The listing builds one solid part. Answer for the finished solid, in the listing's coordinates (mm). A direction names the side the tool comes from. Give positions to 0.01 mm unless a question says otherwise; leave off trailing zeros. Write each loop counter-clockwise with the first axis right and the second up, starting at its lowest first coordinate (ties: lowest second). Pieces come first, ordered by that corner, then holes. Notation, with made-up numbers: (60, -16) - (110, -16) arc R20 cw to (110, 20) - close; hole circle Ø10 at (-17, -13.5). An arc over 180 degrees is marked (long way). Return JSON: item names as keys, results as strings.
Autodesk Inventor part; units mm, degrees
ref_plane "YZ Plane" through (0, 0, 0) normal (1, 0, 0) x (0, 1, 0)
ref_plane "XZ Plane" through (0, 0, 0) normal (0, 1, 0) x (-1, 0, 0)
ref_plane "XY Plane" through (0, 0, 0) normal (0, 0, 1) x (1, 0, 0)
sketch "Skizze1" plane through (0, 0, 0) normal (0, 1, 0) x (-1, 0, 0)
  line L0 (25, -25) -> (-25, -25)
  line L1 (-25, -25) -> (-25, 25)
  line L2 (-25, 25) -> (25, 25)
  line L3 (25, 25) -> (25, -25)
  line L4 (25, -25) -> (-25, 25) construction
  line L5 (-25, -25) -> (25, 25) construction
  point P0 (0, 0)
  dimension "d0" = 50
  dimension "d1" = 50
extrude "Extrusion1" add sketch "Skizze1" along normal blind 6
sketch "Skizze2" plane through (0, 0, 0) normal (0, -1, 0) x (1, 0, 0)
  circle A0 centre (-15.75, 15.75) radius 4.25
  circle A1 centre (15.75, 15.75) radius 4.25
  circle A2 centre (15.75, -15.75) radius 4.25
  circle A3 centre (-15.75, -15.75) radius 4.25
  line L0 (-35, 0) -> (35, 0)
  line L1 (0, 35) -> (0, -35)
  point P0 (0, 0)
  dimension "d4" = 31.5
  dimension "d5" = 31.5
  dimension "d6" = 31.5
  dimension "d7" = 31.5
  dimension "d8" = 15.75
  dimension "d9" = 15.75
  dimension "d10" = 15.75
  dimension "d11" = 15.75
  dimension "d12" = 8.5
  dimension "d13" = 8.5
  dimension "d14" = 8.5
  dimension "d15" = 8.5
extrude "Extrusion2" add sketch "Skizze2" along normal blind 1
sketch "Skizze3" plane through (-15.75, -1, 15.75) normal (0, -1, 0) x (1, 0, 0)
  circle A0 centre (0, 0) radius 4.25
  circle A1 centre (0, 0) radius 1.75
  circle A2 centre (31.5, 0) radius 4.25
  circle A3 centre (31.5, 0) radius 1.75
  circle A4 centre (31.5, -31.5) radius 4.25
  circle A5 centre (31.5, -31.5) radius 1.75
  circle A6 centre (0, -31.5) radius 4.25
  circle A7 centre (0, -31.5) radius 1.75
  point P0 (15.75, -15.75)
  dimension "d18" = 3.5
  dimension "d19" = 3.5
  dimension "d20" = 3.5
  dimension "d21" = 3.5
extrude "Extrusion3" cut sketch "Skizze3" against normal blind 13 contours A1 | A3 | A5 | A7
sketch "Skizze4" plane through (0, 0, 0) normal (0, -1, 0) x (1, 0, 0)
  circle A0 centre (-15, 0) radius 1.5
  circle A1 centre (15, 0) radius 1.5
  line L0 (0, 35) -> (0, -35)
  point P0 (0, 0)
  dimension "d24" = 30
  dimension "d25" = 15
  dimension "d26" = 3
  dimension "d27" = 3
extrude "Extrusion4" cut sketch "Skizze4" against normal blind 13
sketch "Skizze7" plane through (0, 6, 0) normal (0, 1, 0) x (1, 0, 0)
  circle A0 centre (15, 0) radius 1.5
  circle A1 centre (15, 0) radius 3
  circle A2 centre (-15, 0) radius 1.5
  circle A3 centre (-15, 0) radius 3
  point P0 (0, 0)
  dimension "d39" = 6
  dimension "d40" = 6
extrude "Extrusion5" cut sketch "Skizze7" against normal blind 4 contours A0 | A1 | A2 | A3
chamfer "Fase1" distance 1 angle 45 2 edges at (12, 2, 0) (-18, 2, 0)
equation "\"d8\" = 0.5 * d6"
equation "\"d9\" = 0.5 * d7"
equation "\"d10\" = 0.5 * d5"
equation "\"d11\" = 0.5 * d4"
equation "\"d25\" = 0.5 * d24"
properties part number "Lagerhalterung"
Item 1: The mould has two halves that part along Z. Classify faces 4 (the face through (-14.809, 2.451, 17.226)), 5 (the face through (-16, -1, -18)), 6 (the face through (0, 3, -25)): +Z half, -Z half, draft (parallel to the pull), parting line (faces both ways), or undercut.
Answer below:
{"face 4": "undercut", "face 5": "draft", "face 6": "-Z half"}
Item 2: A cutting plane is placed at D-D on z = -15.75. Determine the outline of the cut face in (x, y).
Answer below:
{"outline": "(-25, 0) - (-20, 0) - (-20, -1) - (-17.5, -1) - (-17.5, 6) - (-25, 6) - close; (-14, -1) - (-11.5, -1) - (-11.5, 0) - (11.5, 0) - (11.5, -1) - (14, -1) - (14, 6) - (-14, 6) - close; (17.5, -1) - (20, -1) - (20, 0) - (25, 0) - (25, 6) - (17.5, 6) - close"}
Item 3: Consider L1, parallel to X at y = 4, z = 0; L2, parallel to Z at x = 15, y = 1.25; L3, parallel to Z at x = -15.75, y = 4.25. Determine where each line is inside the solid, lowest interval first.
Answer below:
{"L1": "x = -25 to -18, -12 to 12, 18 to 25", "L2": "z = -25 to -17.33, -14.17 to -1.5, 1.5 to 14.17, 17.33 to 25", "L3": "z = -25 to -17.5, -14 to -2.9, 2.9 to 14, 17.5 to 25"}
Item 4: A cutting plane is placed at A-A on z = 0. Determine the outline of the cut face in (x, y), then the cut area to 3 significant figures.
Answer below:
{"outline": "(-25, 0) - (-16.5, 0) - (-16.5, 2) - (-17, 2) - (-18, 3) - (-18, 6) - (-25, 6) - close; (-13.5, 0) - (13.5, 0) - (13.5, 2) - (13, 2) - (12, 3) - (12, 6) - (-12, 6) - (-12, 3) - (-13, 2) - (-13.5, 2) - close; (16.5, 0) - (25, 0) - (25, 6) - (18, 6) - (18, 3) - (17, 2) - (16.5, 2) - close", "area": "242 mm²"}
Item 5: For faces 1 (the face through (15.522, 2.451, -14.015)), 2 (the face through (12, 5, 0)), 3 (the face through (0, 0, 0)), determine the directions among +Z, -Z, +X, -X, +Y, -Y from which every point of the face is accessible in a straight line to the end or side of a thin tool.
Answer below:
{"face 1": "+Y, -Y", "face 2": "+Y", "face 3": "-Y"}
Item 6: A cutting plane is placed at B-B on y = 4.25. Determine the outline of the cut face in (x, z), then the cut area to 3 significant figures.
Answer below:
{"outline": "(-25, -25) - (25, -25) - (25, 25) - (-25, 25) - close; hole circle Ø6 at (-15, 0); hole circle Ø3.5 at (-15.75, -15.75); hole circle Ø3.5 at (-15.75, 15.75); hole circle Ø6 at (15, 0); hole circle Ø3.5 at (15.75, -15.75); hole circle Ø3.5 at (15.75, 15.75)", "area": "2,400 mm²"}
Item 7: Flat-ended cylindrical pins translate along their axes: P1, Ø5.5, axis at x = 15, z = 0, coming from the -Y side; P2, Ø5.5, axis at x = -15, z = 0, coming from the +Y side. Find the tip coordinate at first contact, or state that the pin passes through.
Answer below:
{"P1": "stops at y = 0", "P2": "stops at y = 2.75"}
Item 8: A cutting plane is placed at C-C on x = 15. Give the number of separate pieces and of enclosed holes in the cut face, then the cut area to 3 significant figures.
Answer below:
{"separate pieces": "4", "enclosed holes": "0", "area": "243 mm²"}
